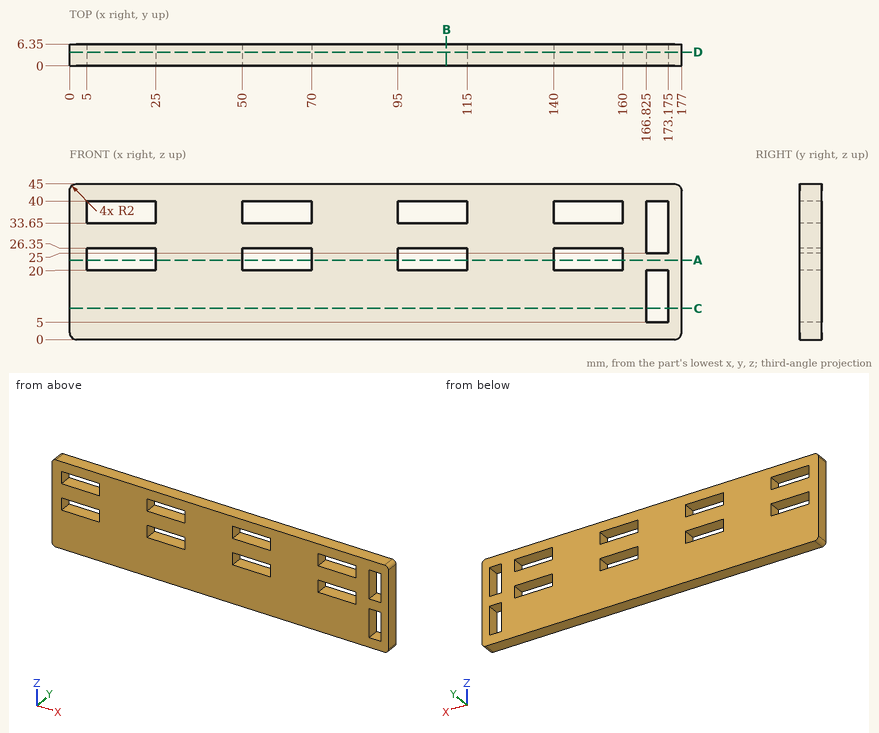
Here's the drawing with two shaded views (mm, measured from the low corner). I have some questions. Coordinates: 2 decimals unless noted, no trailing zeros. Write each loop counter-clockwise with the first axis right and the second up, starting at its lowest first coordinate (ties: lowest second). Pieces come first, ordered by that corner, then holes. Notation, with made-up numbers: (44, 56.5) -> (94, 56.5) arc R20 cw to (94, 67.5) -> close; hole circle Ø11 at (19.5, 38.5). An arc over 180 degrees is marked (long way). One line per question, with ' | ' between items. Start each with the question number.
1. If we section it at C-C (z = 9): Please give me the cut outline in (x, y) (3 decimals).
2. If we section it at A-A (z = 23): Please give me the cut outline in (x, y).
3. If we section it at B-B (x = 109): Please give me the cut outline in (y, z), and give its area (3 significant figures).
4. If we section it at D-D (y = 4): Count the separate pieces of the cut face and the enclosed holes in it, and give its area (3 significant figures).
5. Please list where these lines run through material, in increasing order: line 1 along Z through (x, y) = (141, 5.75); line 2 along X through (y, z) = (4, 34.5) (3 decimals); line 3 along Z through (x, y) = (168, 1.75).
Return value:
1) outline: (0, 0) -> (166.825, 0) -> (166.825, 6.35) -> (0, 6.35) -> close; (173.175, 0) -> (177, 0) -> (177, 6.35) -> (173.175, 6.35) -> close
2) outline: (0, 0) -> (5, 0) -> (5, 6.35) -> (0, 6.35) -> close; (25, 0) -> (50, 0) -> (50, 6.35) -> (25, 6.35) -> close; (70, 0) -> (95, 0) -> (95, 6.35) -> (70, 6.35) -> close; (115, 0) -> (140, 0) -> (140, 6.35) -> (115, 6.35) -> close; (160, 0) -> (177, 0) -> (177, 6.35) -> (160, 6.35) -> close
3) outline: (0, 0) -> (6.35, 0) -> (6.35, 20) -> (0, 20) -> close; (0, 26.35) -> (6.35, 26.35) -> (6.35, 33.65) -> (0, 33.65) -> close; (0, 40) -> (6.35, 40) -> (6.35, 45) -> (0, 45) -> close | area: 205 mm²
4) separate pieces: 1 | enclosed holes: 10 | area: 6,760 mm²
5) line 1: z = 0 to 20, 26.35 to 33.65, 40 to 45 | line 2: x = 0 to 5, 25 to 50, 70 to 95, 115 to 140, 160 to 166.825, 173.175 to 177 | line 3: z = 0 to 5, 20 to 25, 40 to 45
